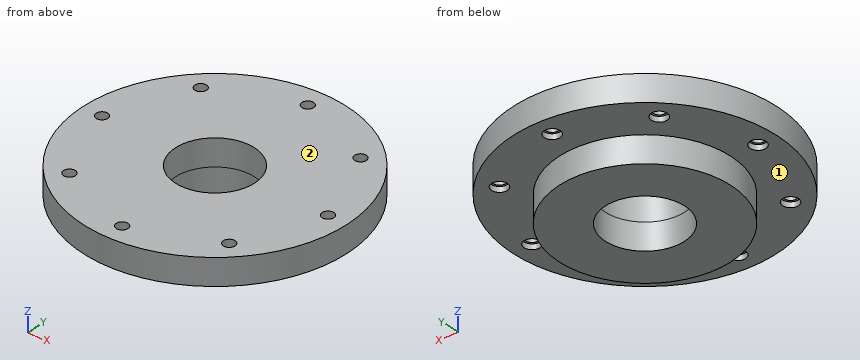
Autodesk Inventor part; units mm, degrees
ref_plane "YZ Plane" through (0, 0, 0) normal (1, 0, 0) x (0, 1, 0)
ref_plane "XZ Plane" through (0, 0, 0) normal (0, 1, 0) x (-1, 0, 0)
ref_plane "XY Plane" through (0, 0, 0) normal (0, 0, 1) x (1, 0, 0)
sketch "Sketch1" plane through (0, 0, 0) normal (0, 0, 1) x (1, 0, 0)
  circle A0 centre (0, 0) radius 50
  circle A1 centre (0, 0) radius 47.5
  circle A2 centre (0, 0) radius 42.5
  circle A3 centre (0, 0) radius 42.5
  circle A4 centre (0, 0) radius 42.5
  circle A5 centre (0, 0) radius 42.5
  circle A6 centre (0, 0) radius 42.5
  circle A7 centre (0, 0) radius 42.5
  circle A8 centre (0, 0) radius 42.5
  circle A9 centre (0, 0) radius 42.5
  point P0 (-42.5, 0)
  point P1 (-30.052, 30.052)
  point P2 (0, 42.5)
  point P3 (30.052, 30.052)
  point P4 (42.5, 0)
  point P5 (30.052, -30.052)
  point P6 (0, -42.5)
  point P7 (-30.052, -30.052)
  dimension "d4" = 85
  dimension "d0" = 100
  dimension "d3" = 95
  dimension "d5" = 360
extrude "Extrusion1" add sketch "Sketch1" along normal blind 10 contours A0 | A1 | A2
hole "Hole1" at (-42.5, 0, 0) at (-30.052, 30.052, 0) at (0, 42.5, 0) at (30.052, 30.052, 0) at (42.5, 0, 0) at (30.052, -30.052, 0) at (0, -42.5, 0) at (-30.052, -30.052, 0) direction (0, 0, 1) diameter 4.4587 depth 10 tip angle 118 counterbore diameter 6 counterbore depth 2
sketch "Sketch2" plane through (0, 0, 10) normal (0, 0, 1) x (1, 0, 0)
  circle A0 centre (0, 0) radius 21
  circle A1 centre (0, 0) radius 15
  dimension "d15" = 42
  dimension "d16" = 30
ref_plane "Work Plane1" through (0, 0, 10) normal (0, 0, 1) x (1, 0, 0)
sketch "Sketch4" plane through (0, 0, 10) normal (0, 0, 1) x (1, 0, 0)
  circle A0 centre (0, 0) radius 15
extrude "Extrusion4" cut sketch "Sketch4" against normal through all
sketch "Sketch5" plane through (0, 0, 0) normal (0, 0, -1) x (-1, 0, 0)
  circle A0 centre (0, 0) radius 32.5
  circle A1 centre (0, 0) radius 15
  point P0 (0, 25)
  dimension "d23" = 25
  dimension "d24" = 65
extrude "Extrusion5" add sketch "Sketch5" along normal blind 10
properties part number "Cover of gearbox"
Check sheet for the modelled part. Datum: model origin and axes. Units: mm. Face numbers are marked on the shaded views. A direction names the side the tool comes from. Coordinates: 2 decimals unless noted, no trailing zeros. Write each loop counter-clockwise with the first axis right and the second up, starting at its lowest first coordinate (ties: lowest second). Pieces come first, ordered by that corner, then holes. Notation, with made-up numbers: M -38.75,33 L 20.25,33 A17 cw 20.25,65 Z; hole C -21.5,41 d6. An arc over 180 degrees is marked long. Answer as CSV lines item,"result".
Q1. Cross-section at A-A (y = 0). Record the boundary of the cut face in (x, z).
Check result:
outline,"M -50,0 L -45.5,0 L -45.5,2 L -44.73,2 L -44.73,10 L -50,10 Z; M -40.27,2 L -39.5,2 L -39.5,0 L -32.5,0 L -32.5,-10 L -15,-10 L -15,10 L -40.27,10 Z; M 15,-10 L 32.5,-10 L 32.5,0 L 39.5,0 L 39.5,2 L 40.27,2 L 40.27,10 L 15,10 Z; M 44.73,2 L 45.5,2 L 45.5,0 L 50,0 L 50,10 L 44.73,10 Z"
Q2. Go/stop test with flat-tipped pins: pin 1 (3 mm diameter, centred on x = -19, y = 34.5, fed in from -Z); pin 2 (5 mm diameter, centred on x = 0, y = -42.5, fed in from -Z); pin 3 (2 mm diameter, centred on y = 24.5, z = 4.5, fed in from -X). Record where each tip stops, or that it passes through.
Check result:
pin 1,"z = 0"
pin 2,"z = 2"
pin 3,"x = -44.13"
Q3. Material ranges on probe 1 along Y at (x, z) = (0, 1.1); probe 2 along X at (y, z) = (1, 4.25); probe 3 along Y at (x, z) = (32, 4.75), recorded low to high. Write a range as from..to.
Check result:
probe 1,"-50..-45.5, -39.5..-15, 15..39.5, 45.5..50"
probe 2,"-49.99..-44.49, -40.51..-14.97, 14.97..40.51, 44.49..49.99"
probe 3,"-38.42..-31.14, -28.97..28.97, 31.14..38.42"
Q4. Cross-section at D-D (z = 5.25). Count the separate pieces of the cut face and the enclosed holes in it, then the cut area to 3 significant figures.
Check result:
separate pieces,"1"
enclosed holes,"9"
area,"7,020 mm^2"
Q5. Set-up check for the marked faces 1 and 2: record each of +Z, -Z, +X, -X, +Y, -Y from which the full face is reachable in a straight line by a thin tool's end or side.
Check result:
face 1,"-Z"
face 2,"+Z, +X, -X, +Y, -Y"
Q6. Cross-section at C-C (y = 42.5). Record the boundary of the cut face in (x, z).
Check result:
outline,"M -26.34,0 L -3,0 L -3,2 L -2.23,2 L -2.23,10 L -26.34,10 Z; M 2.23,2 L 3,2 L 3,0 L 26.34,0 L 26.34,10 L 2.23,10 Z"
